The listing builds one solid part. Answer for the finished solid, in the listing's coordinates (mm). A direction names the side the tool comes from. Coordinates: 2 decimals unless noted, no trailing zeros. Order: outer loops, then holes, each group sorted by start corner. A loop starts at its lowest first (then second) coordinate and runs counter-clockwise, first axis right, second up. Notation, with made-up numbers: (-22, 19) -> (-9, 19) arc R25 ccw to (-9, 36) -> close; hole circle Ø9 at (-7.5, 49). An arc over 180 degrees is marked (long way). Write item = value, one per line.
from build123d import *

# Parameters (mm, degrees)
SKETCH1_R               = 4.025
BOSS_EXTRUDE2_DEPTH     = 36.76
RIDE_SIDE_EXTRUDE_DEPTH = 57.47
LEFT_SIDE_EXTRUDE_DEPTH = 57.47
RIGHT_ARM_EXTRUDE_DEPTH = 10
SERVO_ARM_CUT_DEPTH     = 5
SKETCH18_R              = 3.5
SERVO_HOLE_DEPTH        = 152.7
SKETCH4_R               = 4.025
CUT_EXTRUDE2_DEPTH      = 18.38
SKETCH19_W              = 18.38
SKETCH19_H              = 9
CUT_EXTRUDE3_DEPTH      = 58.64


with BuildPart() as part:
    # Sketch1 → Boss-Extrude2 (new body)
    with BuildSketch(Plane.XY):
        with BuildLine():
            ThreePointArc((16.713283102, 15.01433341), (9.494630573, 8.397245558), (0, 6))
            ThreePointArc((0, 6), (-6, 0), (0, -6))
            Line((0, -6), (45.64, -6))
            ThreePointArc((45.64, -6), (49.882640687, -4.242640687), (51.64, 0))
            Line((51.64, 0), (51.64, 14.475068019))
            Line((51.64, 14.475068019), (59.363014513, 58.27445982))
            ThreePointArc((59.363014513, 58.27445982), (54.496057061, 65.225195404), (47.545321477, 60.358237952))
            Line((47.545321477, 60.358237952), (43.136706696, 35.355741095))
            ThreePointArc((43.136706696, 35.355741095), (36.080788508, 23.1345323), (22.82, 18.308))
            ThreePointArc((22.82, 18.308), (19.350841929, 17.432091905), (16.713283102, 15.01433341))
        make_face()
        Circle(SKETCH1_R, mode=Mode.SUBTRACT)
        with Locations((45.64, 0)):
            Circle(SKETCH1_R, mode=Mode.SUBTRACT)
        with Locations((22.82, 11)):
            Circle(SKETCH1_R, mode=Mode.SUBTRACT)
    extrude(amount=BOSS_EXTRUDE2_DEPTH)

    # Sketch5 → Ride-Side-Extrude (add)
    with BuildSketch(Plane.XY.offset(36.76)):
        with BuildLine():
            Line((55.89005096, 38.578304759), (59.363014513, 58.27445982))
            ThreePointArc((59.363014513, 58.27445982), (54.496057061, 65.225195404), (47.545321477, 60.358237952))
            Line((47.545321477, 60.358237952), (44.072357924, 40.662082891))
            ThreePointArc((44.072357924, 40.662082891), (48.939315376, 33.711347307), (55.89005096, 38.578304759))
        make_face()
    extrude(amount=RIDE_SIDE_EXTRUDE_DEPTH)

    # Sketch7 → Left-Side-Extrude (add)
    with BuildSketch(Plane(origin=(0, 0, 0), x_dir=(-1, 0, 0), z_dir=(0, 0, -1))):
        with BuildLine():
            Line((-44.072357924, 40.662082891), (-47.545321477, 60.358237952))
            ThreePointArc((-47.545321477, 60.358237952), (-54.496057061, 65.225195404), (-59.363014513, 58.27445982))
            Line((-59.363014513, 58.27445982), (-55.89005096, 38.578304759))
            ThreePointArc((-55.89005096, 38.578304759), (-48.939315376, 33.711347307), (-44.072357924, 40.662082891))
        make_face()
    extrude(amount=LEFT_SIDE_EXTRUDE_DEPTH)

    # Sketch16 → Right-Arm-Extrude (add)
    with BuildSketch(Plane.XY.offset(94.23)):
        with BuildLine():
            Line((141.0449767, 80.853531394), (52.412278929, 65.225195404))
            ThreePointArc((52.412278929, 65.225195404), (57.696808682, 63.558989573), (59.363014513, 58.27445982))
            Line((59.363014513, 58.27445982), (58.633475935, 54.137040945))
            Line((58.633475935, 54.137040945), (143.128754832, 69.035838357))
            ThreePointArc((143.128754832, 69.035838357), (147.995712284, 75.986573942), (141.0449767, 80.853531394))
        make_face()
        with BuildLine():
            ThreePointArc((55.89005096, 38.578304759), (98.679190662, 56.18502639), (143.128754832, 69.035838357))
            Line((143.128754832, 69.035838357), (58.633475935, 54.137040945))
            Line((58.633475935, 54.137040945), (55.89005096, 38.578304759))
        make_face()
    right_arm_extrude = extrude(amount=-RIGHT_ARM_EXTRUDE_DEPTH)

    # Sketch17 → Servo-Arm-Cut (cut)
    with BuildSketch(Plane.XY.offset(94.23)):
        with BuildLine():
            Line((141.006923599, 78.796142381), (126.442824066, 74.712393516))
            ThreePointArc((126.442824066, 74.712393516), (124.655768538, 71.871112131), (127.306826897, 69.812389968))
            Line((127.306826897, 69.812389968), (142.389328129, 70.956136704))
            ThreePointArc((142.389328129, 70.956136704), (146.026096778, 75.639277586), (141.006923599, 78.796142381))
        make_face()
    servo_arm_cut = extrude(amount=-SERVO_ARM_CUT_DEPTH, mode=Mode.SUBTRACT)

    # Sketch18 → Servo-hole (cut, through all)
    with BuildSketch(Plane.XY.offset(94.23)):
        with Locations((142.086865766, 74.944684876)):
            Circle(SKETCH18_R)
    servo_hole = extrude(amount=-SERVO_HOLE_DEPTH, mode=Mode.SUBTRACT)

    # Sketch4 → Cut-Extrude2 (cut)
    with BuildSketch(Plane(origin=(0, 0, 9.19), x_dir=(-1, 0, 0), z_dir=(0, 0, -1))):
        with BuildLine():
            Line((-45.64, -6), (0, -6))
            ThreePointArc((0, -6), (6, 0), (0, 6))
            ThreePointArc((0, 6), (-9.494630573, 8.397245558), (-16.713283102, 15.01433341))
            ThreePointArc((-16.713283102, 15.01433341), (-22.82, 18.308), (-28.926716898, 15.01433341))
            ThreePointArc((-28.926716898, 15.01433341), (-36.145369427, 8.397245558), (-45.64, 6))
            ThreePointArc((-45.64, 6), (-51.64, 0), (-45.64, -6))
        make_face()
        with Locations((-45.64, 0)):
            Circle(SKETCH4_R, mode=Mode.SUBTRACT)
        Circle(SKETCH4_R, mode=Mode.SUBTRACT)
        with Locations((-22.82, 11)):
            Circle(SKETCH4_R, mode=Mode.SUBTRACT)
    extrude(amount=-CUT_EXTRUDE2_DEPTH, mode=Mode.SUBTRACT)

    # Sketch19 → Cut-Extrude3 (cut, through all)
    with BuildSketch(Plane(origin=(51.64, 0, 0), x_dir=(0, 0, -1), z_dir=(1, 0, 0))):
        with Locations((-18.38, 4.5)):
            Rectangle(SKETCH19_W, SKETCH19_H)
    extrude(amount=-CUT_EXTRUDE3_DEPTH, mode=Mode.SUBTRACT)

    # Left-Arm Extrude: Right-Arm-Extrude, Servo-Arm-Cut, Servo-hole across plane
    add(right_arm_extrude.mirror(Plane(origin=(0, 0, 18.38), x_dir=(1, 0, 0), z_dir=(0, 0, -1))))
    add(servo_arm_cut.mirror(Plane(origin=(0, 0, 18.38), x_dir=(1, 0, 0), z_dir=(0, 0, -1))), mode=Mode.SUBTRACT)
    add(servo_hole.mirror(Plane(origin=(0, 0, 18.38), x_dir=(1, 0, 0), z_dir=(0, 0, -1))), mode=Mode.SUBTRACT)


solid = part.part
Q1. Section B-B, the plane y = 11 is taken. Give the vertices of the cut face in (x, z) (3 decimals), plus the area to 3 significant figures.
The answers:
outline = (13.229, 0) -> (18.795, 0) -> (18.795, 9.19) -> (13.229, 9.19) -> close; (13.229, 27.57) -> (18.795, 27.57) -> (18.795, 36.76) -> (13.229, 36.76) -> close; (26.845, 0) -> (51.64, 0) -> (51.64, 36.76) -> (26.845, 36.76) -> (26.845, 27.57) -> (32.411, 27.57) -> (32.411, 9.19) -> (26.845, 9.19) -> close
area = 911 mm2
Q2. Section C-C, the plane z = 24.5 is taken. Give the vertices of the cut face in (x, y), plus the area to 3 significant figures.
The answers:
outline = (22.82, 18.31) arc R7.31 cw to (28.93, 15.01) arc R20 ccw to (35.1, 9) -> (51.64, 9) -> (51.64, 14.48) -> (59.36, 58.27) arc R6 ccw to (47.55, 60.36) -> (43.14, 35.36) arc R20.63 cw to start
area = 819 mm2
Q3. Section D-D, the plane y = 25 is taken. Give the vertices of the cut face in (x, z), plus the area to 3 significant figures.
The answers:
outline = (38.03, 0) -> (53.5, 0) -> (53.5, 36.76) -> (38.03, 36.76) -> close
area = 569 mm2
Q4. Each of these flat-tipped pins is pushed along its axis until it touches: pin 1 Ø2 at (y, z) = (34, 74.5) entering from -X; pin 2 Ø10 at (x, y) = (137.5, 72.5) entering from -Z; pin 3 Ø3 at (y, z) = (52, 77.5) entering from -X; pin 4 Ø14 at (x, y) = (11.5, 19) entering from -Z. Where does it stop, or does it pass through?
The answers:
pin_1 = 46.15
pin_2 = -57.47
pin_3 = 45.81
pin_4 = 0
Q5. Section A-A, the plane x = 129.5 is taken. Give the vertices of the cut face in (y, z), plus the area to 3 significant figures.
The answers:
outline = (65.65, -57.47) -> (69.98, -57.47) -> (69.98, -52.47) -> (75.57, -52.47) -> (75.57, -57.47) -> (78.82, -57.47) -> (78.82, -47.47) -> (65.65, -47.47) -> close; (65.65, 84.23) -> (78.82, 84.23) -> (78.82, 94.23) -> (75.57, 94.23) -> (75.57, 89.23) -> (69.98, 89.23) -> (69.98, 94.23) -> (65.65, 94.23) -> close
area = 207 mm2
Q6. Find the intervals of material crossed by line 1 along Y through (x, z) = (0, 5) (3 decimals); line 2 along Z through (x, y) = (84, 55.5); line 3 along Z through (x, y) = (22, -1), in increasing order.
The answers:
line_1 = -6 to -4.025, 4.025 to 6
line_2 = -57.47 to -47.47, 84.23 to 94.23
line_3 = 0 to 9.19, 27.57 to 36.76
Q7. The mould has two halves that part along Y. Classify faces 6 (the face through (3.84, 1.21, 32.1)), 7 (the face through (-6, 0, 32)), 8 (the face through (124.647, 71.922, -55.005)), 9 (the face through (26.24, 17.46, 18.25)): released by +Y, released by -Y, zero draft, split by the parting line, or undercut.
The answers:
face_6 = undercut
face_7 = split by the parting line
face_8 = undercut
face_9 = released by -Y
Q8. A tool of negligible diameter and unlimited length cuts with its end or side. For faces 1 (the face through (49.836, -4.289, 32.101)), 2 (the face through (133.827, 76.783, -55.005)), 3 (the face through (133.827, 76.783, 91.765)), 4 (the face through (31.644, 11.713, 18.251)), 5 (the face through (43, 9, 19)), from which of +Z, -Z, +X, -X, +Y, -Y can it reach the whole face along a straight path? Write none if from no direction.
The answers:
face_1 = +Z, -Z, +X, -Y
face_2 = -Z
face_3 = +Z
face_4 = -X, -Y
face_5 = +X, -X, -Y
